Model file for the job. Use its own axes, mm. Coordinates: 2 decimals unless noted, no trailing zeros. Order: outer loops, then holes, each group sorted by start corner. A loop starts at its lowest first (then second) coordinate and runs counter-clockwise, first axis right, second up. Notation, with made-up numbers: (77, -34.5) - (101, -34.5) arc R26 cw to (101, -12.5) - close; hole circle Ø10 at (61, 1.5). An arc over 180 degrees is marked (long way). Put each result on its own line as item: value. Start each with the question number.
```python
from build123d import *

# Parameters (mm, degrees)
SKETCH1_R                = 0.425
BOSS_EXTRUDE1_DEPTH      = 1.6
LPATTERN2_START          = -0.0125
LPATTERN2_OUTLINE_R      = 0.425
LPATTERN2_DEPTH          = 1.6
SLOTFOOTPRINTS_REF_DEPTH = 0.0001
SLOTFOOTPRINTS_DEPTH     = 0.0001
SKETCH2_R                = 0.8
F_20PIN_MOUNTS_DEPTH     = 71.235674696
SKETCH3_R                = 0.8
F_12PIN_MOUNTS_DEPTH     = 10


# Read off the part's stored shape, not the designer's step: LPattern2
with BuildPart() as part:
    # Sketch1 → Boss-Extrude1 (new body)
    with BuildSketch(Plane(origin=(0, 0, -0.0125), x_dir=(-1, 0, 0), z_dir=(0, 0, -1))):
        with BuildLine():
            Line((35.3, -50), (35.3, -48))
            ThreePointArc((35.3, -48), (35.592893219, -47.292893219), (36.3, -47))
            Line((36.3, -47), (45.8, -47))
            ThreePointArc((45.8, -47), (46.507106781, -46.707106781), (46.8, -46))
            Line((46.8, -46), (46.8, -41.4))
            ThreePointArc((46.8, -41.4), (47.092893219, -40.692893219), (47.8, -40.4))
            Line((47.8, -40.4), (49.3, -40.4))
            Line((49.3, -40.4), (49.3, 39.2))
            Line((49.3, 39.2), (43.2, 45.3))
            Line((43.2, 45.3), (35.500000002, 45.3))
            Line((35.500000002, 45.3), (3.499999998, 45.3))
            Line((3.499999998, 45.3), (-43.2, 45.3))
            Line((-43.2, 45.3), (-49.3, 39.2))
            Line((-49.3, 39.2), (-49.3, -40.4))
            Line((-49.3, -40.4), (-47.8, -40.4))
            ThreePointArc((-47.8, -40.4), (-47.092893219, -40.692893219), (-46.8, -41.4))
            Line((-46.8, -41.4), (-46.8, -46))
            ThreePointArc((-46.8, -46), (-46.507106781, -46.707106781), (-45.8, -47))
            Line((-45.8, -47), (-36.3, -47))
            ThreePointArc((-36.3, -47), (-35.592893219, -47.292893219), (-35.3, -48))
            Line((-35.3, -48), (-35.3, -50))
            Line((-35.3, -50), (35.3, -50))
        make_face()
        with Locations(Location((-21.27, 41.37, 0), (0, 0, 180))):
            Circle(SKETCH1_R, mode=Mode.SUBTRACT)
        with Locations(Location((-23.81, 41.37, 0), (0, 0, 180))):
            Circle(SKETCH1_R, mode=Mode.SUBTRACT)
        with Locations(Location((-22.54, 40.1, 0), (0, 0, 180))):
            Circle(SKETCH1_R, mode=Mode.SUBTRACT)
        with Locations(Location((-13.87, 41.37, 0), (0, 0, 180))):
            Circle(SKETCH1_R, mode=Mode.SUBTRACT)
        with Locations(Location((-23.81, 38.83, 0), (0, 0, 180))):
            Circle(SKETCH1_R, mode=Mode.SUBTRACT)
        with Locations(Location((-16.41, 41.37, 0), (0, 0, 180))):
            Circle(SKETCH1_R, mode=Mode.SUBTRACT)
        with Locations(Location((-15.14, 40.1, 0), (0, 0, 180))):
            Circle(SKETCH1_R, mode=Mode.SUBTRACT)
        with Locations(Location((-21.27, 38.83, 0), (0, 0, 180))):
            Circle(SKETCH1_R, mode=Mode.SUBTRACT)
        with Locations(Location((-28.67, 41.37, 0), (0, 0, 180))):
            Circle(SKETCH1_R, mode=Mode.SUBTRACT)
        with Locations(Location((-31.21, 41.37, 0), (0, 0, 180))):
            Circle(SKETCH1_R, mode=Mode.SUBTRACT)
        with Locations(Location((-16.41, 38.83, 0), (0, 0, 180))):
            Circle(SKETCH1_R, mode=Mode.SUBTRACT)
        with Locations(Location((-29.94, 40.1, 0), (0, 0, 180))):
            Circle(SKETCH1_R, mode=Mode.SUBTRACT)
        with Locations(Location((-31.21, 38.83, 0), (0, 0, 180))):
            Circle(SKETCH1_R, mode=Mode.SUBTRACT)
        with Locations(Location((-28.67, 38.83, 0), (0, 0, 180))):
            Circle(SKETCH1_R, mode=Mode.SUBTRACT)
        with Locations(Location((-13.87, 38.83, 0), (0, 0, 180))):
            Circle(SKETCH1_R, mode=Mode.SUBTRACT)
    extrude(amount=-BOSS_EXTRUDE1_DEPTH)

    # LPattern2 outline → LPattern2 (cut)
    with BuildSketch(Plane.XY.offset(LPATTERN2_START)):
        with Locations((31.21, 31.37)):
            Circle(LPATTERN2_OUTLINE_R)
        with Locations((31.21, 28.83)):
            Circle(LPATTERN2_OUTLINE_R)
        with Locations((29.94, 30.1)):
            Circle(LPATTERN2_OUTLINE_R)
        with Locations((28.67, 28.83)):
            Circle(LPATTERN2_OUTLINE_R)
        with Locations((28.67, 31.37)):
            Circle(LPATTERN2_OUTLINE_R)
        with Locations((16.41, 31.37)):
            Circle(LPATTERN2_OUTLINE_R)
        with Locations((23.81, 31.37)):
            Circle(LPATTERN2_OUTLINE_R)
        with Locations((23.81, 28.83)):
            Circle(LPATTERN2_OUTLINE_R)
        with Locations((22.54, 30.1)):
            Circle(LPATTERN2_OUTLINE_R)
        with Locations((21.27, 28.83)):
            Circle(LPATTERN2_OUTLINE_R)
        with Locations((21.27, 31.37)):
            Circle(LPATTERN2_OUTLINE_R)
        with Locations((16.41, 28.83)):
            Circle(LPATTERN2_OUTLINE_R)
        with Locations((15.14, 30.1)):
            Circle(LPATTERN2_OUTLINE_R)
        with Locations((13.87, 28.83)):
            Circle(LPATTERN2_OUTLINE_R)
        with Locations((13.87, 31.37)):
            Circle(LPATTERN2_OUTLINE_R)
    extrude(amount=LPATTERN2_DEPTH, mode=Mode.SUBTRACT)

    # thermalContacts_lower → slotFootprints_REF (cut)
    with BuildSketch(Plane(origin=(0, 0, -0.0125), x_dir=(-1, 0, 0), z_dir=(0, 0, -1))):
        Polygon((47, 35.5), (47, -41.5), (59.827263463, -41.5), (59.827263463, 47), (41.5, 47), (41.5, 41.5), (41.5, 35.5), align=None)
        Polygon((-47, 35.5), (-47, -41.5), (-56.192158269, -41.5), (-56.192158269, 47), (-41.5, 47), (-41.5, 41.5), (-41.5, 35.5), align=None)
    extrude(amount=-SLOTFOOTPRINTS_REF_DEPTH, mode=Mode.SUBTRACT)

    # thermalContacts_upper → slotFootprints (cut)
    with BuildSketch(Plane.XY.offset(1.5875)):
        Polygon((-47, 35.5), (-47, -41.5), (-56.192158269, -41.5), (-56.192158269, 47), (-41.5, 47), (-41.5, 41.5), (-41.5, 35.5), align=None)
        Polygon((47, 35.5), (47, -41.5), (59.827263463, -41.5), (59.827263463, 47), (41.5, 47), (41.5, 41.5), (41.5, 35.5), align=None)
    extrude(amount=-SLOTFOOTPRINTS_DEPTH, mode=Mode.SUBTRACT)

    # Sketch2 → 20pin_mounts (cut, through all)
    with BuildSketch(Plane.XY.offset(1.5875)):
        with Locations((-33.775, 38.472296419)):
            Circle(SKETCH2_R)
        with Locations((-17.925, 38.472296419)):
            Circle(SKETCH2_R)
        with Locations((-17.925, 28.472296419)):
            Circle(SKETCH2_R)
        with Locations((-33.775, 28.472296419)):
            Circle(SKETCH2_R)
        with BuildLine():
            Line((-35.775, 45.3), (-35.775, 43.8))
            ThreePointArc((-35.775, 43.8), (-35.482106781, 43.092893219), (-34.775, 42.8))
            Line((-34.775, 42.8), (-16.925, 42.8))
            ThreePointArc((-16.925, 42.8), (-16.217893218, 43.092893219), (-15.925, 43.8))
            Line((-15.925, 43.8), (-15.925, 45.3))
            Line((-15.925, 45.3), (-35.775, 45.3))
        make_face()
    extrude(amount=-F_20PIN_MOUNTS_DEPTH, mode=Mode.SUBTRACT)

    # Sketch3 → 12pin_mounts (cut)
    with BuildSketch(Plane(origin=(0, 0, -0.0125), x_dir=(-1, 0, 0), z_dir=(0, 0, -1))):
        with Locations((5.390000006, 42.3)):
            Circle(SKETCH3_R)
        with Locations((-5.379999994, 42.3)):
            Circle(SKETCH3_R)
        with Locations((42.3, 5.379999994)):
            Circle(SKETCH3_R)
        with Locations((42.3, -5.390000006)):
            Circle(SKETCH3_R)
        with Locations((5.390000006, -42.303202712)):
            Circle(SKETCH3_R)
        with Locations((-5.379999994, -42.303202712)):
            Circle(SKETCH3_R)
        with Locations((-42.3, -5.390000006)):
            Circle(SKETCH3_R)
        with Locations((-42.3, 5.379999994)):
            Circle(SKETCH3_R)
        with BuildLine():
            Line((-49.3, 7.379999994), (-48, 7.379999994))
            ThreePointArc((-48, 7.379999994), (-47.292893219, 7.087106775), (-47, 6.379999994))
            Line((-47, 6.379999994), (-47, -6.390000006))
            ThreePointArc((-47, -6.390000006), (-47.292893219, -7.097106787), (-48, -7.390000006))
            Line((-48, -7.390000006), (-49.3, -7.390000006))
            Line((-49.3, -7.390000006), (-49.3, 7.379999994))
        make_face()
        with BuildLine():
            Line((48, 7.379999994), (49.3, 7.379999994))
            Line((49.3, 7.379999994), (49.3, -7.390000006))
            Line((49.3, -7.390000006), (48, -7.390000006))
            ThreePointArc((48, -7.390000006), (47.292893219, -7.097106787), (47, -6.390000006))
            Line((47, -6.390000006), (47, 6.379999994))
            ThreePointArc((47, 6.379999994), (47.292893219, 7.087106775), (48, 7.379999994))
        make_face()
        with BuildLine():
            Line((-6.379999994, -46.203202712), (6.390000006, -46.203202712))
            ThreePointArc((6.390000006, -46.203202712), (7.097106787, -46.496095931), (7.390000006, -47.203202712))
            Line((7.390000006, -47.203202712), (7.390000006, -50))
            Line((7.390000006, -50), (-7.379999994, -50))
            Line((-7.379999994, -50), (-7.379999994, -47.203202712))
            ThreePointArc((-7.379999994, -47.203202712), (-7.087106775, -46.496095931), (-6.379999994, -46.203202712))
        make_face()
    extrude(amount=-F_12PIN_MOUNTS_DEPTH, mode=Mode.SUBTRACT)


solid = part.part
```
Item 1: Slice it at B-B, the plane x = 40. Give the cut face in (y, z), plus the area to 3 significant figures.
Item 2: Wall check: line 1 along Y through (x, z) = (-18, 0.7); line 2 along Y through (x, z) = (31.21, 1.1) (3 decimals); line 3 along Y through (x, z) = (-42.3, 1.3). Give the ranges that are in metal, low to high.
Item 3: Flat gauge pins, fed straight in: pin 1 Ø0.8 at (y, z) = (-43.5, 1) entering from +X; pin 2 Ø0.8 at (x, z) = (38.5, 1) entering from -Y. Where does each tip first touch, or does it go through?
Item 4: Slice it at C-C, the plane z = 0.35. Give the number of separate pieces and of enclosed holes in the cut face, plus the area to 3 significant figures.
Item 5: Slice it at A-A, the plane y = 0.5. Give the cut face in (x, z).
Here are the results:
1. outline: (-47, -0.01) - (45.3, -0.01) - (45.3, 1.59) - (-47, 1.59) - close
1. area: 148 mm^2
2. line 1: y = -50 to 27.68, 29.27 to 37.68, 39.27 to 42.8
2. line 2: y = -50 to 28.405, 29.255 to 30.945, 31.795 to 38.405, 39.255 to 40.945, 41.795 to 45.3
2. line 3: y = -47 to -6.19, -4.59 to 4.58, 6.18 to 45.3
3. pin 1: stops at x = 46.8
3. pin 2: stops at y = -47
4. separate pieces: 1
4. enclosed holes: 42
4. area: 9,030 mm^2
5. outline: (-47, -0.01) - (47, -0.01) - (47, 1.59) - (-47, 1.59) - close
